Could you check a few things on this model? Use its own coordinates, in mm. A direction names the side the tool comes from. Give positions to 0.01 mm unless a question says otherwise; leave off trailing zeros. Order: outer loops, then holes, each group sorted by start corner. A loop starts at its lowest first (then second) coordinate and runs counter-clockwise, first axis right, second up.
(1) If we mould it in two halves opening along Z, with no side actions, what happens to faces 6 (the flat face through (-5, -26.67, -5)), 7 (the flat face through (64.866, -13.148, -5.403)), 8 (the flat face through (-5, -13, -9.286))? For each: released by +Z, released by -Z, zero draft, split by the parting line, or undercut.
(2) Imagine slicing it at C-C, the plane z = -3.5. Write out the boundary of the cut face in (x, y).
(3) Imagine slicing it at B-B, the plane y = -4. Write out the boundary of the cut face in (x, z).
(4) Imagine slicing it at D-D, the plane z = 6.5. Write out the boundary of the cut face in (x, y).
(5) Will these pins go through, and if not, where does the flat tip stop? pin 1 (2 mm diameter, centred on y = -4.5, z = 11, fed in from -X); pin 2 (3 mm diameter, centred on y = -11, z = 3.5, fed in from -X); pin 3 (8 mm diameter, centred on y = -7, z = 3.5, fed in from +X).
(6) On a 3-axis mill with a long thin cutter (end or side, diameter ignored), from which of +Z, -Z, +X, -X, +Y, -Y can I reach the whole of each face in a straight line? I mean faces 1 (the flat face through (-3, -13, 16.627)), 2 (the flat face through (-72.007, -13.148, 12.744)), 3 (the flat face through (-5, -25.4, 4)), 4 (the flat face through (64.826, -13.148, 12.634)), 5 (the flat face through (-5, 0, 4)). Say none if no direction works.
(7) If I drill on probe 1 along X at (y, z) = (-10.5, 2.25); probe 2 along Y at (x, z) = (-39.5, 8.5); probe 3 along X at (y, z) = (-25.5, 10.25), over which ranges is the centre line in solid material (lowest first)?
(8) Imagine slicing it at A-A, the plane x = 11. Write out the boundary of the cut face in (y, z), then the cut area to 3 significant figures.
from build123d import *

# Parameters (mm, degrees)
F1_DEPTH = 25.4
F3_DEPTH = 1.27
F4_DEPTH = 1.27


with BuildPart() as f1:
    # F0 (on Front) → F1 (new body)
    with BuildSketch(Plane.XZ):
        Polygon((66.279829, 16.627325), (-73.420171, 16.627325), (-70.553358, 8.750822), (-70.553358, -1.409178), (-73.420171, -9.285682), (66.279829, -9.285682), (63.413016, -1.409178), (63.413016, 8.750822), align=None)
    extrude(amount=F1_DEPTH)

    # F2 (on face) → F3 (join)
    with BuildSketch(Plane.XZ.offset(25.4)):
        Polygon((-73.420171, 16.627325), (-70.553358, 8.750822), (63.413016, 8.750822), (66.279829, 16.627325), align=None)
    extrude(amount=F3_DEPTH)

    # F2 (on face) → F4 (join)
    with BuildSketch(Plane.XZ.offset(25.4)):
        Polygon((63.413016, -1.409178), (-70.553358, -1.409178), (-73.420171, -9.285682), (66.279829, -9.285682), align=None)
    extrude(amount=F4_DEPTH)


solid = f1.part
Answer block:
1. face 6: zero draft
1. face 7: undercut
1. face 8: released by -Z
2. outline: (-71.31, -26.67) - (64.17, -26.67) - (64.17, 0) - (-71.31, 0) - close
3. outline: (-73.42, -9.29) - (66.28, -9.29) - (63.41, -1.41) - (63.41, 8.75) - (66.28, 16.63) - (-73.42, 16.63) - (-70.55, 8.75) - (-70.55, -1.41) - close
4. outline: (-70.55, -25.4) - (63.41, -25.4) - (63.41, 0) - (-70.55, 0) - close
5. pin 1: stops at x = -71.74
5. pin 2: stops at x = -70.55
5. pin 3: stops at x = 63.41
6. face 1: +Z, +X, -X, +Y, -Y
6. face 2: -X, +Y, -Y
6. face 3: +X, -X, -Y
6. face 4: +X, +Y, -Y
6. face 5: +Z, -Z, +X, -X, +Y
7. probe 1: x = -70.55 to 63.41
7. probe 2: y = -25.4 to 0
7. probe 3: x = -71.1 to 63.96
8. outline: (-26.67, -9.29) - (0, -9.29) - (0, 16.63) - (-26.67, 16.63) - (-26.67, 8.75) - (-25.4, 8.75) - (-25.4, -1.41) - (-26.67, -1.41) - close
8. area: 678 mm2
